Could you check a few things on this model? Use its own coordinates, in mm. A direction names the side the tool comes from. Give positions to 0.01 mm unless a question says otherwise; leave off trailing zeros. Order: outer loops, then holes, each group sorted by start corner. A loop starts at its lowest first (then second) coordinate and runs counter-clockwise, first axis right, second up. Notation, with made-up numbers: M -31,62.25 L -4,62.25 A27 cw -4,90.25 Z; hole C -0.5,86 d11. An arc over 180 degrees is marked long. Answer in a Markdown table with one row per item. Add a question column.
Autodesk Inventor part; units mm, degrees
ref_plane "Work Plane1" through (0, 13, 0) normal (0, 1, 0) x (1, 0, 0)
ref_plane "YZ Plane" through (0, 0, 0) normal (1, 0, 0) x (0, 1, 0)
ref_plane "XZ Plane" through (0, 0, 0) normal (0, 1, 0) x (-1, 0, 0)
sketch "Sketch1" plane through (0, 0, 0) normal (0, 1, 0) x (-1, 0, 0)
  line L0 (-130, 30) -> (130, 30)
  line L1 (130, 30) -> (130, -30)
  line L2 (130, -30) -> (-130, -30)
  line L3 (-130, -30) -> (-130, 30)
  line L4 (-130, 30) -> (130, -30) construction
  line L5 (130, 30) -> (-130, -30) construction
  line L6 (-30, -130) -> (-30, 130)
  line L7 (-30, 130) -> (30, 130)
  line L8 (30, 130) -> (30, -130)
  line L9 (30, -130) -> (-30, -130)
  line L10 (-30, -130) -> (30, 130) construction
  line L11 (-30, 130) -> (30, -130) construction
  line L12 (130, -30) -> (-130, -30)
  line L13 (-130, -30) -> (-130, 30)
  line L14 (-130, 30) -> (130, 30)
  line L15 (130, 30) -> (130, -30)
  line L16 (130, -30) -> (-130, 30) construction
  line L17 (-130, -30) -> (130, 30) construction
  line L18 (30, 130) -> (30, -130)
  line L19 (30, -130) -> (-30, -130)
  line L20 (-30, -130) -> (-30, 130)
  line L21 (-30, 130) -> (30, 130)
  line L22 (30, 130) -> (-30, -130) construction
  line L23 (30, -130) -> (-30, 130) construction
  arc A0 (130, -30) -> (130, 30) centre (0, 0) ccw
  line L24 (-130, 0) -> (-107.5, 0) construction
  circle A1 centre (0, 0) radius 107.5
  circle A2 centre (0, 0) radius 92.5
  line L25 (-30, 87.5) -> (-30, 77)
  line L26 (-30, 77) -> (-38, 77)
  circle A3 centre (0, 0) radius 99.5
  line L27 (-38, 77) -> (-38, 91.9579)
  line L28 (-87.5, 30) -> (-77, 30)
  line L29 (-77, 30) -> (-77, 38)
  line L30 (-77, 38) -> (-91.9579, 38)
  line L31 (-34, 77) -> (-34, 81) construction
  line L32 (-77, 34) -> (-81, 34) construction
  line L33 (-81, 34) -> (-81, 30) construction
  point P0 (-30, 30)
  point P1 (-30, 30)
  point P2 (-30, 77)
  point P3 (-30, 103.2291)
  point P4 (-103.2291, 30)
  point P5 (-77, 30)
  dimension "d1" = 260
  dimension "d2" = 60
  dimension "d5" = 360
  dimension "d7" = 22.5
  dimension "d8" = 15
  dimension "d9" = 10.5
  dimension "d10" = 8
  dimension "d11" = 8
  dimension "d12" = 10.5
  dimension "d13" = 8
  dimension "d14" = 4
  dimension "d15" = 4
  dimension "d16" = 4
extrude "Extrusion1" add sketch "Sketch1" along normal blind 26 contours A2 L30 L29 L0 | L0 A3 L30 A2 | L0 A1 L6 A3 | L27 A3 L6 A2 | A2 L6 L26 L27
fillet "Fillet1" radius 2 4 edges at (38, 13, 91.9579) (91.9579, 13, 38) (77, 13, 38) (38, 13, 77)
hole "Hole1" at (34, 0, 81) at (81, 0, 34) direction (0, 1, 0) diameter 4.2 depth 6
ref_plane "Work Plane1" through (0, 13, 0) normal (0, 1, 0) x (1, 0, 0)
mirror "Mirror1" about plane through (0, 13, 0) normal (0, 1, 0) of "Hole1"
fillet "Fillet2" radius 1.5 2 edges at (103.2291, 13, 30) (30, 13, 103.2291)
equation "\"d9\" = d12"
equation "\"d10\" = d11"
equation "\"d13\" = d11"
equation "\"d14\" = 0.5 * d11"
equation "\"d15\" = 0.5 * d11"
equation "\"d16\" = 0.5 * d11"
properties part number "Side Wall"
1. For faces 4 (the flat face through (33, 13, 77)), 5 (the cylindrical face through (32.722, 22.958, 82.666)), 6 (the flat face through (34, 6, 81)), 7 (the flat face through (84, 13, 38)), 8 (the flat face through (38, 13, 84)), which set-ups out of +Z, -Z, +X, -X, +Y, -Y let a thin tool reach every point of the face, with its end or its side?
2. Suppose I cut it at B-B on z = 85.5. List the corners of the cut face in (x, y) for me.
3. If I drill on line 1 along X through (y, z) = (4.3, 81); line 2 along Z through (x, y) = (81.5, 2.5), over which ranges is the centre line in solid material (lowest first)? Write a range as [from, to].
4. Thinking about a two-plate mould opening in X: for faces 1 (the cylindrical face through (102.431, 13.182, 30.627)), 2 (the flat face through (81, 20, 34)), 3 (the flat face through (72, 26, 69)), which applies, pulls with the +X half, pulls with the -X half, needs draft (parallel to the pull), parting line crosses it, or undercut?
5. Will these pins go through, and if not, where does the flat tip stop? P1, Ø3, axis at x = 69, y = 5.5, coming from the +Z side; P2, Ø3, axis at y = 10.5, z = 64.5, coming from the -X side; P3, Ø2.5, axis at x = 81, z = 34, coming from the +Y side; P4, Ø5.5, axis at x = 34, z = 81, coming from the +Y side.
6. Suppose I cut it at A-A on y = 21. List the corners of the cut face in (x, z) for me.
7. Suppose I cut it at C-C on x = 81. List the corners of the cut face in (y, z) for me, plus the area to 3 significant figures.
8. Suppose I cut it at D-D on y = 8.75. List the corners of the cut face in (x, z) for me, plus the area to 3 significant figures.
Findings below:
| question | item | result |
|---|---|---|
| 1 | face 4 | -Z, -X, +Y, -Y |
| 1 | face 5 | +Y |
| 1 | face 6 | -Y |
| 1 | face 7 | -X, +Y, -Y |
| 1 | face 8 | -Z, +Y, -Y |
| 2 | outline | M 30,0 L 38,0 L 38,26 L 30,26 Z; M 50.89,0 L 65.16,0 L 65.16,26 L 50.89,26 Z |
| 3 | line 1 | [30, 31.9], [36.1, 38], [57.79, 70.68] |
| 3 | line 2 | [30, 31.96], [36.04, 38], [57.08, 70.1] |
| 4 | face 1 | pulls with the +X half |
| 4 | face 2 | undercut |
| 4 | face 3 | needs draft |
| 5 | P1 | z = 83.67 |
| 5 | P2 | x = 74.46 |
| 5 | P3 | y = 20 |
| 5 | P4 | y = 26 |
| 6 | outline | M 30,77 L 36,77 A2 ccw 38,79 L 38,88.92 A2 cw 40.82,90.74 A99.5 cw 90.74,40.82 A2 cw 88.92,38 L 79,38 A2 ccw 77,36 L 77,30 L 101.21,30 A1.5 ccw 102.64,31.95 A107.5 ccw 31.95,102.64 A1.5 ccw 30,101.21 Z; hole C 34,81 d4.2; hole C 81,34 d4.2 |
| 7 | outline | M 0,30 L 26,30 L 26,31.9 L 20,31.9 L 20,36.1 L 26,36.1 L 26,38 L 0,38 L 0,36.1 L 6,36.1 L 6,31.9 L 0,31.9 Z; M 0,57.79 L 26,57.79 L 26,70.68 L 0,70.68 Z |
| 7 | area | 493 mm2 |
| 8 | outline | M 30,77 L 36,77 A2 ccw 38,79 L 38,88.92 A2 cw 40.82,90.74 A99.5 cw 90.74,40.82 A2 cw 88.92,38 L 79,38 A2 ccw 77,36 L 77,30 L 101.21,30 A1.5 ccw 102.64,31.95 A107.5 ccw 31.95,102.64 A1.5 ccw 30,101.21 Z |
| 8 | area | 1,080 mm2 |
